from build123d import *

# Parameters (mm, degrees)
SKETCH1_W           = 304.8
SKETCH1_H           = 127
BOSS_EXTRUDE1_DEPTH = 101.6
CUT_EXTRUDE2_DEPTH  = 95.25
SKETCH3_W           = 289.56
SKETCH3_H           = 111.76
BOSS_EXTRUDE2_DEPTH = 6.35
SKETCH5_R           = 15.24
CUT_EXTRUDE4_DEPTH  = 372.316040041
FILLET2_R           = 5.08
SKETCH6_R           = 16.51
CUT_EXTRUDE5_DEPTH  = 2.54


with BuildPart() as part:
    # Sketch1 → Boss-Extrude1 (new body)
    with BuildSketch(Plane.XY):
        Rectangle(SKETCH1_W, SKETCH1_H)
    extrude(amount=BOSS_EXTRUDE1_DEPTH)

    # 3DSketch1 → Cut-Extrude2 (cut)
    with BuildSketch(Plane(origin=(144.78, 55.88, 101.6), x_dir=(-0.9329231300425795, -0.36007559405152184, 0), z_dir=(0, 0, 1))):
        Polygon((0, 0), (270.137221535, -104.263489014), (310.379269926, 0), (40.242048391, 104.263489014), align=None)
    extrude(amount=-CUT_EXTRUDE2_DEPTH, mode=Mode.SUBTRACT)

    # Sketch3 → Boss-Extrude2 (add)
    with BuildSketch(Plane.XY.offset(101.6)):
        with BuildLine():
            Line((-103.259510137, 89.837120171), (103.425046446, 89.837120171))
            ThreePointArc((103.425046446, 89.837120171), (193.262166618, 0), (103.425046446, -89.837120171))
            Line((103.425046446, -89.837120171), (-103.259510137, -89.837120171))
            ThreePointArc((-103.259510137, -89.837120171), (-193.096630308, 0), (-103.259510137, 89.837120171))
        make_face()
        Rectangle(SKETCH3_W, SKETCH3_H, mode=Mode.SUBTRACT)
    extrude(amount=-BOSS_EXTRUDE2_DEPTH)

    # Sketch5 → Cut-Extrude4 (cut, through all)
    with BuildSketch(Plane.ZY.offset(152.4)):
        with Locations(Location((48.26, 17.78, 0), (0, 0, 270))):
            Circle(SKETCH5_R)
    extrude(amount=-CUT_EXTRUDE4_DEPTH, mode=Mode.SUBTRACT)

    # Fillet2
    fillet2_edges = [part.edges().sort_by_distance(p)[0] for p in [
        (0, -55.88, 101.6),
    ]]
    fillet(fillet2_edges, radius=FILLET2_R)

    # Sketch6 → Cut-Extrude5 (cut)
    with BuildSketch(Plane(origin=(152.4, 0, 0), x_dir=(0, 0, -1), z_dir=(1, 0, 0))):
        with Locations((-48.26, 17.78)):
            Circle(SKETCH6_R)
    cut_extrude5 = extrude(amount=-CUT_EXTRUDE5_DEPTH, mode=Mode.SUBTRACT)

    # Mirror1: Cut-Extrude5 across plane
    add(cut_extrude5.mirror(Plane(origin=(0, 0, 0), x_dir=(0, 0, 1), z_dir=(1, 0, 0))), mode=Mode.SUBTRACT)


solid = part.part
The listing builds one solid part. Answer for the finished solid, in the listing's coordinates (mm). A direction names the side the tool comes from. Give positions to 0.01 mm unless a question says otherwise; leave off trailing zeros. Write each loop counter-clockwise with the first axis right and the second up, starting at its lowest first coordinate (ties: lowest second). Pieces come first, ordered by that corner, then holes.
Item 1: Section A-A, the plane z = 48.26 is taken. Write down the section's boundary in (x, y).
Item 2: Section C-C, the plane z = 26 is taken. Write down the section's boundary in (x, y).
Item 3: Section D-D, the plane x = 140.5 is taken. Write down the section's boundary in (y, z), plus the area to 3 significant figures.
Item 4: Section B-B, the plane y = 11.5 is taken. Write down the section's boundary in (x, z).
Item 5: Determine the mould class of faces 1 (the cylindrical face through (-147.36, 21.08, 33.38)), 2 (the cylindrical face through (193.24, 1.98, 98.47)), 3 (the flat face through (-144.78, -2, 55)), 4 (the cylindrical face through (-193.075, -1.975, 98.469)) for opening direction X: released by +X, released by -X, zero draft, split by the parting line, or undercut.
Item 6: Which of the six approach directions +Z, -Z, +X, -X, +Y, -Y give full straight-line access (tool end or side, diameter ignored) to faces 5 (the flat face through (-152.4, -1, 47)), 6 (the flat face through (-2, -63.5, 47)), 7 (the cylindrical face through (-151.1, 22.7, 32.5)), 8 (the flat face through (144.78, -3, 55)), 9 (the cylindrical face through (151.1, 22.7, 32.5))?
Item 7: Find the intervals of material crossed by line 1 along Y through (x, z) = (-141, 58); line 2 along X through (y, z) = (-10, 34.5); line 3 along Y through (x, z) = (148, 48), in increasing order.
Item 8: Flat-ended cylindrical pins translate along their axes: P1, Ø10, axis at x = -141, z = 77, coming from the +Y side; P2, Ø1, axis at x = 49.5, y = 45.5, coming from the +Z side; P3, Ø10, axis at x = -7.5, y = 30.5, coming from the -Z side. Find the tip coordinate at first contact, or state that the pin passes through.
Completed:
1. outline: (-152.4, -63.5) - (152.4, -63.5) - (152.4, 1.27) - (149.86, 1.27) - (149.86, 2.54) - (144.78, 2.54) - (144.78, -55.88) - (-144.78, -55.88) - (-144.78, 2.54) - (-149.86, 2.54) - (-149.86, 1.27) - (-152.4, 1.27) - close; (-152.4, 34.29) - (-149.86, 34.29) - (-149.86, 33.02) - (-144.78, 33.02) - (-144.78, 55.88) - (144.78, 55.88) - (144.78, 33.02) - (149.86, 33.02) - (149.86, 34.29) - (152.4, 34.29) - (152.4, 63.5) - (-152.4, 63.5) - close
2. outline: (-152.4, -63.5) - (152.4, -63.5) - (152.4, 63.5) - (-152.4, 63.5) - close; hole (-144.78, -55.88) - (144.78, -55.88) - (144.78, 55.88) - (-144.78, 55.88) - close
3. outline: (-81.83, 95.25) - (-63.5, 95.25) - (-63.5, 0) - (63.5, 0) - (63.5, 95.25) - (81.83, 95.25) - (81.83, 101.6) - (55.88, 101.6) - (55.88, 6.35) - (-55.88, 6.35) - (-55.88, 96.52) arc R5.08 ccw to (-60.96, 101.6) - (-81.83, 101.6) - close
3. area: 2,490 mm2
4. outline: (-192.36, 95.25) - (-152.4, 95.25) - (-152.4, 63.53) - (-149.86, 63.53) - (-149.86, 62.15) - (-144.78, 62.15) - (-144.78, 101.6) - (-192.36, 101.6) - close; (-152.4, 0) - (152.4, 0) - (152.4, 32.99) - (149.86, 32.99) - (149.86, 34.37) - (144.78, 34.37) - (144.78, 6.35) - (-144.78, 6.35) - (-144.78, 34.37) - (-149.86, 34.37) - (-149.86, 32.99) - (-152.4, 32.99) - close; (144.78, 62.15) - (149.86, 62.15) - (149.86, 63.53) - (152.4, 63.53) - (152.4, 95.25) - (192.52, 95.25) - (192.52, 101.6) - (144.78, 101.6) - close
5. face 1: zero draft
5. face 2: released by +X
5. face 3: undercut
5. face 4: released by -X
6. face 5: -Z, -X, +Y, -Y
6. face 6: -Z, +X, -X, -Y
6. face 7: -X
6. face 8: +Z
6. face 9: +X
7. line 1: y = -63.5 to -55.88, 55.88 to 63.5
7. line 2: x = -152.4 to -144.78, 144.78 to 152.4
7. line 3: y = -63.5 to 2.54, 33.02 to 63.5
8. P1: stops at y = 63.5
8. P2: stops at z = 6.35
8. P3: stops at z = 0
